Geometry check sheet. Reference: drawing and pictorial views, mm from the part's lowest x, y, z. Coordinates: 2 decimals unless noted, no trailing zeros. Loops run counter-clockwise (first coordinate to the right, second up) from the corner with the lowest first, then second, coordinate; pieces in that order, holes last. Notation, with made-up numbers: (79.5, 53.5) -> (95.5, 53.5) arc R11 ccw to (95.5, 70.5) -> close; hole circle Ø6 at (60.5, 88). An arc over 180 degrees is marked (long way). Answer as a JSON object with one key per item and string values. Group by question number.
Q1. Cross-section at C-C on x = 12.45. Record the boundary of the cut face in (y, z) (3 decimals), and give its area (3 significant figures).
Q2. Cross-section at A-A on y = 8. Record the boundary of the cut face in (x, z) (3 decimals), and give its area (3 significant figures).
Q3. Scan lines: L1, parallel to Y at x = 12.45, z = 1.75 (3 decimals); L2, parallel to Z at x = 11.75, y = 9; L3, parallel to X at y = 24.25, z = 1.45. Record each from-to range of solid material in increasing order.
Q4. Gauge pin test, flat end, axial feed: pin 1 Ø0.9 at (x, y) = (13, 7.5) entering from +Z. Record the tip position at first contact, or that the pin passes through.
Q5. Cross-section at B-B on z = 1.75. Record the boundary of the cut face in (x, y) (3 decimals), and give its area (3 significant figures).
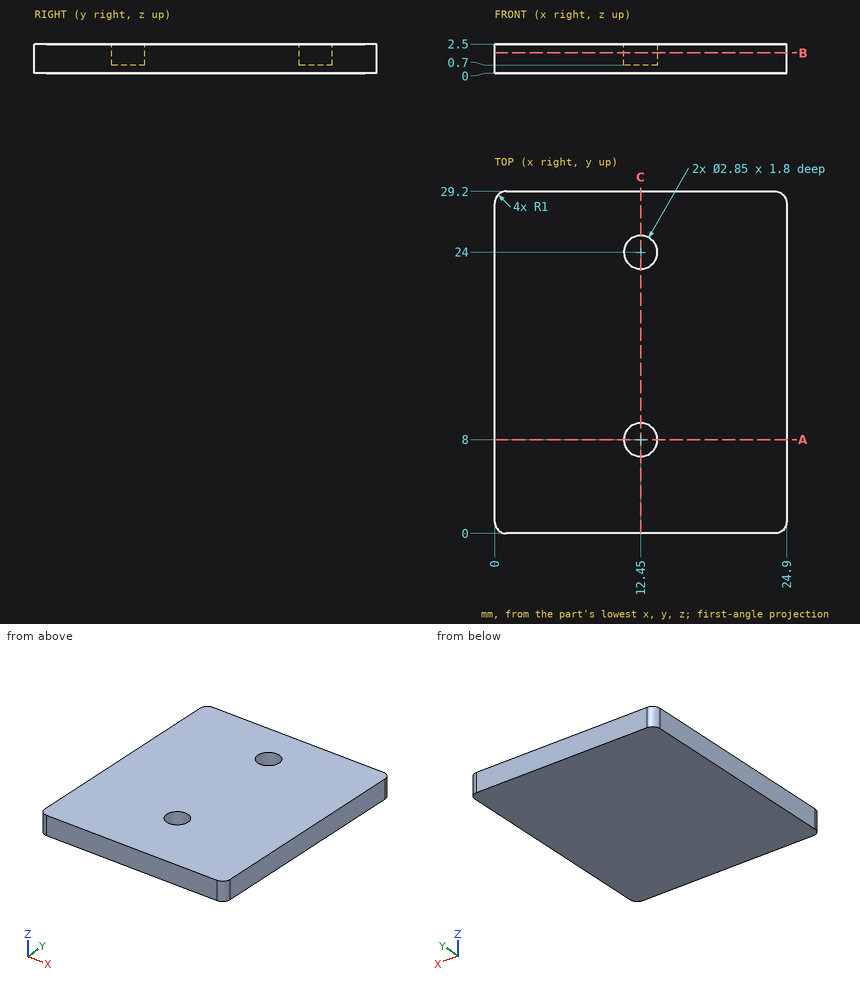
Computed values:
{
 "1": {"outline": "(0, 0) -> (29.2, 0) -> (29.2, 2.5) -> (25.425, 2.5) -> (25.425, 0.7) -> (22.575, 0.7) -> (22.575, 2.5) -> (9.425, 2.5) -> (9.425, 0.7) -> (6.575, 0.7) -> (6.575, 2.5) -> (0, 2.5) -> close", "area": "62.7 mm²"},
 "2": {"outline": "(0, 0) -> (24.9, 0) -> (24.9, 2.5) -> (13.875, 2.5) -> (13.875, 0.7) -> (11.025, 0.7) -> (11.025, 2.5) -> (0, 2.5) -> close", "area": "57.1 mm²"},
 "3": {"L1": "y = 0 to 6.575, 9.425 to 22.575, 25.425 to 29.2", "L2": "z = 0 to 0.7", "L3": "x = 0 to 11.05, 13.85 to 24.9"},
 "4": {"pin 1": "stops at z = 0.7"},
 "5": {"outline": "(0, 1) arc R1 ccw to (1, 0) -> (23.9, 0) arc R1 ccw to (24.9, 1) -> (24.9, 28.2) arc R1 ccw to (23.9, 29.2) -> (1, 29.2) arc R1 ccw to (0, 28.2) -> close; hole circle Ø2.85 at (12.45, 8); hole circle Ø2.85 at (12.45, 24)", "area": "713 mm²"}
}
